CAD build for the part. Positions are in the model's coordinates, mm. A direction names the side the tool comes from. Coordinates: 2 decimals unless noted, no trailing zeros. Loops run counter-clockwise (first coordinate to the right, second up) from the corner with the lowest first, then second, coordinate; pieces in that order, holes last. Notation, with made-up numbers: (-17.75, 72) -> (28.25, 72) arc R35 cw to (28.25, 107) -> close; hole circle Ø7 at (43.5, -0.5). An arc over 180 degrees is marked (long way). Write item = value, one per line. Start each with the question number.
(1) Drill centre lines: line 1 (Z direction, x = -90.5, y = 31.5); line 2 (X direction, y = 101, z = -31); line 3 (Y direction, x = -137, z = -23.5). Where is each one in solid material? Low to high. Write a range as from..to.
(2) Band-saw the part on C-C (z = -62). Write the cut outline in (x, y), and give its area (3 significant figures).
(3) Tool access for faces 1 (the face through (-95, 125, -73)), 2 (the face through (0, 76, -1)), 3 (the face through (-76, 5, -1)): list every direction of +Z, -Z, +X, -X, +Y, -Y with a clear straight run to the whole face (end or side of a thin tool).
(4) Band-saw the part on B-B (y = 126.5). Write the cut outline in (x, z).
(5) Band-saw the part on A-A (y = 76.5). Write the cut outline in (x, z).
(6) Pull direction Z, two halves, no side cores. Call faces 4 (the face through (-76, 76, 75)), 5 (the face through (-74, 79, -70)), 6 (the face through (-75, 150, 72)): +Z half, -Z half, draft (parallel to the pull), parting line (faces both ways), or undercut.
(7) Band-saw the part on D-D (x = -50.5). Write the cut outline in (y, z), and give its area (3 significant figures).
(8) Flat gauge pins, fed straight in: P1, Ø6, axis at y = 86, z = 33, coming from the +X side; P2, Ø6, axis at x = -96.5, z = 39.5, coming from the +Y side; P3, Ø4, axis at x = -76.5, z = -72.5, coming from the +Y side. Where does each tip first touch, or does it go through?
Autodesk Inventor part; units mm, degrees
ref_plane "YZ Plane" through (0, 0, 0) normal (1, 0, 0) x (0, 1, 0)
ref_plane "XZ Plane" through (0, 0, 0) normal (0, 1, 0) x (-1, 0, 0)
ref_plane "XY Plane" through (0, 0, 0) normal (0, 0, 1) x (1, 0, 0)
sketch "Sketch1" plane through (0, 0, 0) normal (0, 0, 1) x (1, 0, 0)
  line L0 (0, 0) -> (-150, 0)
  line L1 (-150, 0) -> (-150, 150)
  line L2 (-150, 150) -> (0, 150)
  line L3 (0, 150) -> (0, 0)
  dimension "d0" = 150
  dimension "d1" = 150
extrude "Extrusion1" add sketch "Sketch1" along normal mid plane 150
sketch "Sketch2" plane through (-150, 150, 75) normal (0, 1, 0) x (1, 0, 0)
  line L0 (150, 0) -> (0, 0)
  line L1 (150, 150) -> (150, 0)
  line L2 (0, 0) -> (150, 0)
  line L3 (150, 0) -> (150, 150)
  line L4 (150, 150) -> (0, 150)
  line L5 (0, 150) -> (0, 0)
  line L6 (5, 5) -> (145, 5)
  line L7 (145, 5) -> (145, 145)
  line L8 (145, 145) -> (5, 145)
  line L9 (5, 145) -> (5, 5)
  point P0 (150, 75)
  dimension "d4" = 5
  dimension "d5" = 5
  dimension "d6" = 5
  dimension "d7" = 5
extrude "Extrusion2" cut sketch "Sketch2" against normal blind 145 contours L9 L8 L7 L6
sketch "Sketch3" plane through (-150, 150, 75) normal (0, 1, 0) x (1, 0, 0)
  line L0 (0, 0) -> (150, 0)
  line L1 (150, 0) -> (150, 150)
  line L2 (150, 150) -> (0, 150)
  line L3 (0, 150) -> (0, 0)
  line L4 (150, 150) -> (0, 150)
  line L5 (75, 150) -> (75, 0) construction
  line L6 (55, 150) -> (55, 145)
  line L7 (5, 145) -> (145, 145) construction
  line L8 (55, 145) -> (95, 145)
  line L9 (95, 150) -> (95, 145)
  point P0 (150, 75)
  dimension "d10" = 20
  dimension "d11" = 20
extrude "Extrusion3" cut sketch "Sketch3" against normal blind 50 contours L2 L9 L8 L6
properties part number "electronics bay"
Findings below:
q1.line_1 = -75..-70, 70..75
q1.line_2 = -150..-145, -5..0
q1.line_3 = 0..5
q2.outline = (-150, 0) -> (0, 0) -> (0, 150) -> (-5, 150) -> (-5, 5) -> (-145, 5) -> (-145, 150) -> (-150, 150) -> close
q2.area = 2,200 mm²
q3.face_1 = -Z, +Y
q3.face_2 = +Z, -Z, +X, +Y, -Y
q3.face_3 = +Y
q4.outline = (-150, -75) -> (-95, -75) -> (-95, -70) -> (-145, -70) -> (-145, 70) -> (-5, 70) -> (-5, -70) -> (-55, -70) -> (-55, -75) -> (0, -75) -> (0, 75) -> (-150, 75) -> close
q5.outline = (-150, -75) -> (0, -75) -> (0, 75) -> (-150, 75) -> close; hole (-145, -70) -> (-5, -70) -> (-5, 70) -> (-145, 70) -> close
q6.face_4 = +Z half
q6.face_5 = undercut
q6.face_6 = draft
q7.outline = (0, -75) -> (150, -75) -> (150, -70) -> (5, -70) -> (5, 70) -> (150, 70) -> (150, 75) -> (0, 75) -> close
q7.area = 2,200 mm²
q8.P1 = 0
q8.P2 = 5
q8.P3 = 100
